Could you check a few things on this model? Use its own coordinates, in mm. A direction names the side the tool comes from. Round coordinates to 2 decimals unless told otherwise and drop trailing zeros. Order: outer loops, then holes, each group sorted by start corner. A loop starts at its lowest first (then second) coordinate and runs counter-clockwise, first axis right, second up.
```python
from build123d import *

# Parameters (mm, degrees)
SKETCH1_W               = 20.8
SKETCH1_H               = 12.7
BOSS_EXTRUDE1_DEPTH     = 6.4
BOSS_EXTRUDE2_DEPTH     = 1.5
SKETCH5_R               = 1.35
CUT_EXTRUDE1_DEPTH      = 21.181984541
SKETCH9_W               = 12.6
SKETCH9_H               = 1.3
BOSS_EXTRUDE4_DEPTH     = 1.5
SKETCH10_W              = 0.5
SKETCH10_H              = 15.3
BOSS_EXTRUDE5_DEPTH     = 0.2
LPATTERN1_COUNT         = 5
LPATTERN1_PITCH         = 2.54
MIRROR2_COPY_1_SKETCH_W = 0.5
MIRROR2_COPY_1_SKETCH_H = 15.3
MIRROR2_COPY_1_DEPTH    = 0.2
MIRROR2_COPY_2_SKETCH_W = 0.5
MIRROR2_COPY_2_SKETCH_H = 15.3
MIRROR2_COPY_2_DEPTH    = 0.2
MIRROR2_COPY_3_SKETCH_W = 0.5
MIRROR2_COPY_3_SKETCH_H = 15.3
MIRROR2_COPY_3_DEPTH    = 0.2
MIRROR2_COPY_4_SKETCH_W = 0.5
MIRROR2_COPY_4_SKETCH_H = 15.3
MIRROR2_COPY_4_DEPTH    = 0.2
SKETCH12_R              = 0.5
BOSS_EXTRUDE6_DEPTH     = 25


with BuildPart() as part:
    # Sketch1 → Boss-Extrude1 (new body)
    with BuildSketch(Plane(origin=(0, 0, 0), x_dir=(1, 0, 0), z_dir=(0, 1, 0))):
        Rectangle(SKETCH1_W, SKETCH1_H)
    extrude(amount=BOSS_EXTRUDE1_DEPTH)

    # Sketch3 → Boss-Extrude2 (add)
    with BuildSketch(Plane.XZ):
        Polygon((-10.4, 10.95), (-6.6, 10.95), (-6.6, 6.35), (15, 6.35), (15, -6.35), (-6.6, -6.35), (-6.6, -10.95), (-10.4, -10.95), align=None)
    extrude(amount=BOSS_EXTRUDE2_DEPTH)

    # Sketch5 → Cut-Extrude1 (cut, through all)
    with BuildSketch(Plane.XZ.offset(1.5)):
        with Locations(Location((-8.5, 8.95, 0), (0, 0, 270))):
            Circle(SKETCH5_R)
        with Locations(Location((13, 4.45, 0), (0, 0, 270))):
            Circle(SKETCH5_R)
    cut_extrude1 = extrude(amount=-CUT_EXTRUDE1_DEPTH, mode=Mode.SUBTRACT)

    # Mirror3: Cut-Extrude1 across plane
    add(cut_extrude1.mirror(Plane.XY), mode=Mode.SUBTRACT)

    # Sketch11 → Revolve1 (revolve)
    with BuildSketch(Plane(origin=(0, 3.2, 0), x_dir=(-1, 0, 0), z_dir=(0, -1, 0)), mode=Mode.PRIVATE) as revolve1_sk:
        Polygon((-10.4, 1.5), (-10.4, 3.6), (-23.8, 3.6), (-27.7, 2.65), (-38.3, 2.65), (-38.3, 1.5), align=None)
    revolve(revolve1_sk.sketch.rotate(Axis((10.4, 3.2, -1.5), (1, 0, 0)), 180), axis=Axis((10.4, 3.2, -1.5), (1, 0, 0)))

    # Sketch9 → Boss-Extrude4 (add)
    with BuildSketch(Plane(origin=(0, 2.665, 0), x_dir=(-1, 0, 0), z_dir=(0, -1, 0))):
        with Locations((-2.9, -7)):
            Rectangle(SKETCH9_W, SKETCH9_H)
    boss_extrude4 = extrude(amount=-BOSS_EXTRUDE4_DEPTH)

    # Sketch10 → Boss-Extrude5 (add)
    with BuildSketch(Plane(origin=(0, 4.165, 0), x_dir=(1, 0, 0), z_dir=(0, 1, 0))):
        with Locations((7.87, -14)):
            Rectangle(SKETCH10_W, SKETCH10_H)
    boss_extrude5 = extrude(amount=BOSS_EXTRUDE5_DEPTH)

    # LPattern1: Boss-Extrude5 ×5
    with Locations(*[(-i * LPATTERN1_PITCH, 0, 0) for i in range(1, LPATTERN1_COUNT)]):
        add(boss_extrude5)

    # Mirror2: Boss-Extrude4, Boss-Extrude5 across plane
    add(boss_extrude4.mirror(Plane.XY))
    add(boss_extrude5.mirror(Plane.XY))

    # Mirror2 copy 1 sketch → Mirror2 copy 1 (add)
    with BuildSketch(Plane(origin=(-2.54, 4.165, 0), x_dir=(1, 0, 0), z_dir=(0, 1, 0))):
        with Locations((7.87, 14)):
            Rectangle(MIRROR2_COPY_1_SKETCH_W, MIRROR2_COPY_1_SKETCH_H)
    extrude(amount=MIRROR2_COPY_1_DEPTH)

    # Mirror2 copy 2 sketch → Mirror2 copy 2 (add)
    with BuildSketch(Plane(origin=(-5.08, 4.165, 0), x_dir=(1, 0, 0), z_dir=(0, 1, 0))):
        with Locations((7.87, 14)):
            Rectangle(MIRROR2_COPY_2_SKETCH_W, MIRROR2_COPY_2_SKETCH_H)
    extrude(amount=MIRROR2_COPY_2_DEPTH)

    # Mirror2 copy 3 sketch → Mirror2 copy 3 (add)
    with BuildSketch(Plane(origin=(-7.62, 4.165, 0), x_dir=(1, 0, 0), z_dir=(0, 1, 0))):
        with Locations((7.87, 14)):
            Rectangle(MIRROR2_COPY_3_SKETCH_W, MIRROR2_COPY_3_SKETCH_H)
    extrude(amount=MIRROR2_COPY_3_DEPTH)

    # Mirror2 copy 4 sketch → Mirror2 copy 4 (add)
    with BuildSketch(Plane(origin=(-10.16, 4.165, 0), x_dir=(1, 0, 0), z_dir=(0, 1, 0))):
        with Locations((7.87, 14)):
            Rectangle(MIRROR2_COPY_4_SKETCH_W, MIRROR2_COPY_4_SKETCH_H)
    extrude(amount=MIRROR2_COPY_4_DEPTH)

    # Sketch12 → Boss-Extrude6 (add)
    with BuildSketch(Plane(origin=(38.3, 0, 0), x_dir=(0, 0, -1), z_dir=(1, 0, 0))):
        with Locations((1.5, 3.2)):
            Circle(SKETCH12_R)
    extrude(amount=BOSS_EXTRUDE6_DEPTH)


solid = part.part
```
Q1. For faces 4 (the flat face through (-3.4, 3, 7)), 5 (the flat face through (-7.6, 0, 7.7)), 6 (the flat face through (9.2, 3, -7)), 7 (the flat face through (2, 4.165, 7)), 8 (the cylindrical face through (17.194, 1.118, -1.773)), which set-ups out of +Z, -Z, +X, -X, +Y, -Y let a thin tool reach every point of the face, with its end or its side?
Q2. Imagine slicing it at C-C, the plane z = -8.95. Please give me the cut outline in (x, y) (3 decimals), then the cut area to 3 significant figures.
Q3. Imagine slicing it at A-A, the plane z = -16.5. Please give me the cut outline in (x, y) (3 decimals), then the cut area to 3 significant figures.
Q4. We'd pull the mould along Y, two halves only. Please class faces 1 (the flat face through (13, 0, 0)), 2 (the flat face through (4, 4.165, 7)), 3 (the flat face through (-0.3, 2.5, -6.35)): released by +Y, released by -Y, zero draft, split by the parting line, or undercut.
Q5. For P1, Ø12, axis at x = 3, z = 15.5, coming from the +Y side (3 decimals); P2, Ø2, axis at x = -8.5, z = 8.95, coming from the -Y side, each with a flat end and sliding along its axis, tell me the tip position at first contact or that it passes through.
Q6. I need wall thicknesses on L1, parallel to X at y = -1, z = 8.95; L2, parallel to X at y = 5.5, z = -5; L3, parallel to Z at x = 6, y = 4. Which ranges of each line are inside material? Lowest first, please.
Q7. Imagine slicing it at B-B, the plane x = -8.5. Please give me the cut outline in (y, z), then the cut area to 3 significant figures.
Q8. Imagine slicing it at D-D, the plane x = 13. Please give me the cut outline in (y, z).
Filled in:
1. face 4: +Z, -X, +Y, -Y
1. face 5: +Z, +X, -X, +Y
1. face 6: -Z, +X, +Y, -Y
1. face 7: +Z, +Y
1. face 8: +X
2. outline: (-10.4, -1.5) - (-9.85, -1.5) - (-9.85, 0) - (-10.4, 0) - close; (-7.15, -1.5) - (-6.6, -1.5) - (-6.6, 0) - (-7.15, 0) - close; (-2.54, 4.165) - (-2.04, 4.165) - (-2.04, 4.365) - (-2.54, 4.365) - close; (0, 4.165) - (0.5, 4.165) - (0.5, 4.365) - (0, 4.365) - close; (2.54, 4.165) - (3.04, 4.165) - (3.04, 4.365) - (2.54, 4.365) - close; (5.08, 4.165) - (5.58, 4.165) - (5.58, 4.365) - (5.08, 4.365) - close; (7.62, 4.165) - (8.12, 4.165) - (8.12, 4.365) - (7.62, 4.365) - close
2. area: 2.15 mm2
3. outline: (-2.54, 4.165) - (-2.04, 4.165) - (-2.04, 4.365) - (-2.54, 4.365) - close; (0, 4.165) - (0.5, 4.165) - (0.5, 4.365) - (0, 4.365) - close; (2.54, 4.165) - (3.04, 4.165) - (3.04, 4.365) - (2.54, 4.365) - close; (5.08, 4.165) - (5.58, 4.165) - (5.58, 4.365) - (5.08, 4.365) - close; (7.62, 4.165) - (8.12, 4.165) - (8.12, 4.365) - (7.62, 4.365) - close
3. area: 0.500 mm2
4. face 1: undercut
4. face 2: released by +Y
4. face 3: zero draft
5. P1: stops at y = 4.365
5. P2: passes through
6. L1: x = -10.4 to -9.85, -7.15 to -6.6
6. L2: x = -10.4 to 10.4
6. L3: z = -7.65 to 7.65
7. outline: (-1.5, -10.95) - (0, -10.95) - (0, -10.3) - (-1.5, -10.3) - close; (-1.5, -7.6) - (0, -7.6) - (0, -6.35) - (6.4, -6.35) - (6.4, 6.35) - (0, 6.35) - (0, 7.6) - (-1.5, 7.6) - close; (-1.5, 10.3) - (0, 10.3) - (0, 10.95) - (-1.5, 10.95) - close
7. area: 106 mm2
8. outline: (-1.5, -6.35) - (0, -6.35) - (0, -5.8) - (-1.5, -5.8) - close; (-1.5, -3.1) - (0, -3.1) - (0, 3.1) - (-1.5, 3.1) - close; (-1.5, 5.8) - (0, 5.8) - (0, 6.35) - (-1.5, 6.35) - close; circle Ø4.2 at (3.2, -1.5)
